from build123d import *

# Parameters (mm, degrees)
FILLET1_R = 0.508


with BuildPart() as part:
    # Sketch1 → Revolve1 (revolve)
    with BuildSketch(Plane.XY, mode=Mode.PRIVATE) as revolve1_sk:
        with BuildLine():
            Line((0, 5.08), (0, 0))
            ThreePointArc((0, 0), (1.261643301, -0.667825992), (2.159, -1.778))
            Line((2.159, -1.778), (2.159, -3.048))
            Line((2.159, -3.048), (3.175, -3.048))
            Line((3.175, -3.048), (3.175, -0.9652))
            Line((3.175, -0.9652), (2.159, -0.9652))
            Line((2.159, -0.9652), (2.159, 2.4892))
            Line((2.159, 2.4892), (3.445798114, 2.4892))
            Line((3.445798114, 2.4892), (3.445798114, 2.8956))
            ThreePointArc((3.445798114, 2.8956), (2.039922057, 4.487890303), (0, 5.08))
        make_face()
    revolve(revolve1_sk.sketch.rotate(Axis((0, 5.379452632, 0), (0, -1, 0)), 90), axis=Axis((0, 5.379452632, 0), (0, -1, 0)))

    # Fillet1
    fillet1_edges = [part.edges().sort_by_distance(p)[0] for p in [
        (0, -3.048, -3.175),
    ]]
    fillet(fillet1_edges, radius=FILLET1_R)


solid = part.part
Can you work these out from the model? Positions are in its coordinate system, mm. A direction names the side the tool comes from. Give positions to 0.01 mm unless a question says otherwise; leave off trailing zeros. Write each loop counter-clockwise with the first axis right and the second up, starting at its lowest first coordinate (ties: lowest second). Pieces come first, ordered by that corner, then holes. Notation, with made-up numbers: M 46,47.5 L 90,47.5 A18 ccw 90,73.5 Z; hole C -19,56 d8. An arc over 180 degrees is marked long. Answer in a Markdown table with one row per item. Add a question column.
Item 1: On a 3-axis mill with a long thin cutter (end or side, diameter ignored), from which of +Z, -Z, +X, -X, +Y, -Y can I reach the whole of each face in a straight line? I mean faces 3 (the flat face through (0.72, 2.489, -2.25)), 4 (the cylindrical face through (3.364, 2.695, -0.747)), 5 (the cylindrical face through (-2.14, -2.42, -0.28)). Say none if no direction works.
Item 2: Imagine slicing it at B-B, the plane y = 3.25. Write out the boundary of the cut face in (x, z).
Item 3: Imagine slicing it at A-A, the plane y = 4.75. Write out the boundary of the cut face in (x, z), plus the area to 3 significant figures.
Item 4: Please list where these lines run through material, in increasing order: L1, parallel to Y at x = -2.25, z = 0; L2, parallel to Y at x = 2.25, z = -1; L3, parallel to X at y = -0.75, z = 1.
Item 5: We'd pull the mould along Y, two halves only. Please class faces 1 (the cylindrical face through (1.93, -1.74, -2.52)), 2 (the cylindrical face through (-2.14, 0.79, -0.28)): released by +Y, released by -Y, zero draft, split by the parting line, or undercut.
Item 6: For pin 1 Ø1.5 at (y, z) = (3, -2.5) entering from +X; pin 2 Ø1.9 at (x, z) = (1.5, -1) entering from +Y; pin 3 Ø1.5 at (y, z) = (-0.5, -0.5) entering from +X (3 decimals), each with a flat end and sliding along its axis, tell me the tip position at first contact or that it passes through.
Evaluation:
| question | item | result |
|---|---|---|
| 1 | face 3 | none |
| 1 | face 4 | +Y, -Y |
| 1 | face 5 | -Y |
| 2 | outline | C 0,0 d6.51 |
| 3 | outline | C 0,0 d3.1 |
| 3 | area | 7.56 mm² |
| 4 | L1 | y = -3.05 to -0.97, 2.49 to 4.34 |
| 4 | L2 | y = -3.05 to -0.97, 2.49 to 4.18 |
| 4 | L3 | x = -1.91 to -0.92, 0.92 to 1.91 |
| 5 | face 1 | zero draft |
| 5 | face 2 | undercut |
| 6 | pin 1 | stops at x = 2.96 |
| 6 | pin 2 | stops at y = 4.98 |
| 6 | pin 3 | stops at x = 3.175 |
